Here's how the part is built. I have some questions about the finished solid (model axes, mm). A direction names the side the tool comes from. Coordinates: 2 decimals unless noted, no trailing zeros. Loops run counter-clockwise (first coordinate to the right, second up) from the corner with the lowest first, then second, coordinate; pieces in that order, holes last. Notation, with made-up numbers: M -35,60 L 0,60 A22 ccw 0,95 Z; hole C 38,84 d4. An arc over 180 degrees is marked long. Use one line per item in the form item = value. Start each with the question number.
(1) On a 3-axis mill with a long thin cutter (end or side, diameter ignored), from which of +Z, -Z, +X, -X, +Y, -Y can I reach the whole of each face in a straight line? I mean faces 1 (the flat face through (17.5, 0, -25)), 2 (the flat face through (0, 17.5, -25)), 3 (the flat face through (0, 17.5, 2025)), 4 (the flat face through (0, -17.5, -25)). Say none if no direction works.
(2) Imagine slicing it at A-A, the plane y = -1. Please give me the cut outline in (x, z).
(3) Will these pins go through, and if not, where does the flat tip stop? P1, Ø17.5, axis at y = -2, z = 2023.5, coming from the +X side; P2, Ø4, axis at x = 23.5, y = 27, coming from the +Z side; P3, Ø17.5, axis at y = -3.5, z = -24, coming from the -X side.
(4) Please list where this line runs through material, in increasing order: L1, parallel to Z at x = -25, y = -30.
```python
from build123d import *

# Parameters (mm, degrees)
F0_W     = 75
F0_H     = 75
F1_DEPTH = 2000
F2_W     = 35
F2_H     = 35
F4_DEPTH = 50
F3_W     = 35
F3_H     = 35
F5_DEPTH = 50


with BuildPart() as f1:
    # F0 (on Top) → F1 (new body)
    with BuildSketch(Plane.XY):
        Rectangle(F0_W, F0_H)
    extrude(amount=F1_DEPTH)

    # F2 (on face) → F4 (join)
    with BuildSketch(Plane(origin=(0, 0, 0), x_dir=(1, 0, 0), z_dir=(0, 0, -1))):
        Rectangle(F2_W, F2_H)
    extrude(amount=F4_DEPTH)

    # F3 (on face) → F5 (join)
    with BuildSketch(Plane.XY.offset(2000)):
        Rectangle(F3_W, F3_H)
    extrude(amount=F5_DEPTH)


solid = f1.part
```
Answer:
q1.face_1 = -Z, +X, +Y, -Y
q1.face_2 = -Z, +X, -X, +Y
q1.face_3 = +Z, +X, -X, +Y
q1.face_4 = -Z, +X, -X, -Y
q2.outline = M -37.5,0 L -17.5,0 L -17.5,-50 L 17.5,-50 L 17.5,0 L 37.5,0 L 37.5,2000 L 17.5,2000 L 17.5,2050 L -17.5,2050 L -17.5,2000 L -37.5,2000 Z
q3.P1 = 17.5
q3.P2 = 2000
q3.P3 = -17.5
q4.L1 = 0 to 2000
